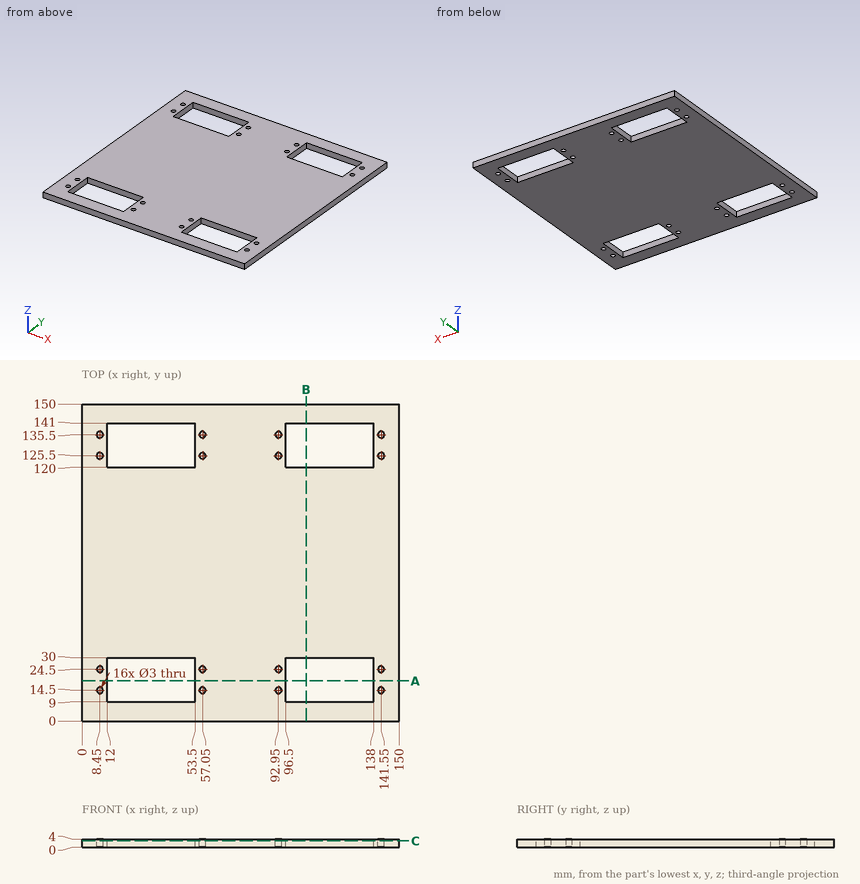
The figure shows three views and two pictorial views of one solid part (mm, origin at its lowest corner). Answer the questions. Give positions to 0.01 mm unless a question says otherwise; leave off trailing zeros. Write each loop counter-clockwise with the first axis right and the second up, starting at its lowest first coordinate (ties: lowest second). Pieces come first, ordered by that corner, then holes. Notation, with made-up numbers: M 19,49 L 54,49 A19 cw 54,69 Z; hole C 14.5,48.25 d5. An arc over 180 degrees is marked long. Write each question's results on one line, items separated by ' | '.
Q1. Section C-C, the plane z = 3.15 is taken. Count the separate pieces of the cut face and the enclosed holes in it, then the cut area to 3 significant figures.
Output values:
separate pieces: 1 | enclosed holes: 20 | area: 18,900 mm2
Q2. Section B-B, the plane x = 106 is taken. Write down the section's boundary in (y, z), then the cut area to 3 significant figures.
Output values:
outline: M 0,0 L 9,0 L 9,4 L 0,4 Z; M 30,0 L 120,0 L 120,4 L 30,4 Z; M 141,0 L 150,0 L 150,4 L 141,4 Z | area: 432 mm2
Q3. Consider L1, parallel to Y at x = 104.5, z = 1.05; L2, parallel to X at y = 12.5, z = 3.6; L3, parallel to Y at x = 8.45, z = 1.25. Determine where each line is inside the solid, lowest interval first. Write a range as from..to.
Output values:
L1: 0..9, 30..120, 141..150 | L2: 0..12, 53.5..96.5, 138..150 | L3: 0..13, 16..23, 26..124, 127..134, 137..150
Q4. Section A-A, the plane y = 19 is taken. Write down the section's boundary in (x, z), then the cut area to 3 significant figures.
Output values:
outline: M 0,0 L 12,0 L 12,4 L 0,4 Z; M 53.5,0 L 96.5,0 L 96.5,4 L 53.5,4 Z; M 138,0 L 150,0 L 150,4 L 138,4 Z | area: 268 mm2
